Could you check a few things on this model? Use its own coordinates, in mm. Face numbers are marked on the shaded views. A direction names the side the tool comes from. Give positions to 0.01 mm unless a question says otherwise; leave off trailing zeros. Loops run counter-clockwise (first coordinate to the right, second up) from the corner with the lowest first, then second, coordinate; pieces in that order, holes last. Notation, with made-up numbers: (-23, 57) - (-10, 57) arc R16 cw to (-10, 61) - close; hole circle Ø3 at (7, 55.25). An arc over 180 degrees is marked (long way). One line per item, written item: value. Start each with the question number.
Q1. I'm going to push flat-ended pins straight in: P1, Ø10, axis at y = 13, z = 50, coming from the +X side; P2, Ø5, axis at y = 62.5, z = 36.5, coming from the -X side; P3, Ø13, axis at x = -20, z = 52.49, coming from the +Y side. Where does each tip first touch, or does it pass through?
Q2. I want a section at B-B (z = 22). Please give me the cut outline in (x, y), then the cut area to 3 significant figures.
Q3. If we mould it in two halves opening along Y, with no side actions, what happens to the marked faces 4, 5 and 6? For each: released by +Y, released by -Y, zero draft, split by the parting line, or undercut.
Q4. For the marked faces 1, 2 and 3, which set-ups out of +Z, -Z, +X, -X, +Y, -Y let a thin tool reach every point of the face, with its end or its side?
Q5. I want a section at D-D (z = 51). Please give me the cut outline in (x, y), then the cut area to 3 significant figures.
Q6. I want a section at C-C (x = -20). Please give me the cut outline in (y, z).
Q7. If I drill on line 1 (Y direction, x = -53.5, z = 24.5); line 2 (Z direction, x = 16, y = 14.5); line 3 (X direction, y = 10.5, z = 38), over which ranges is the centre line in solid material (lowest first)? Write a range as from..to.
Q8. I want a section at A-A (x = -68). Please give me the cut outline in (y, z), then the cut area to 3 significant figures.
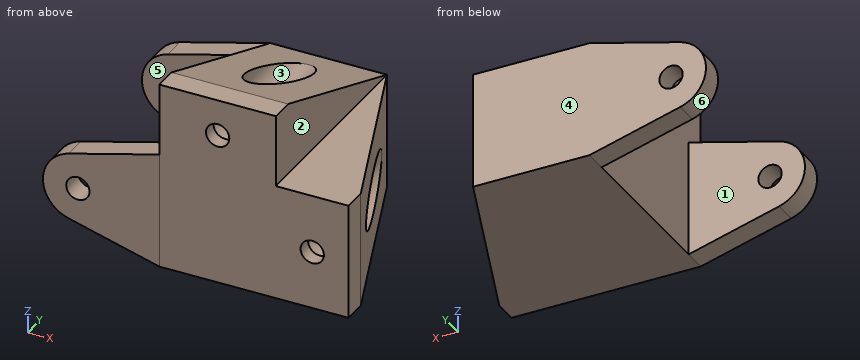
```python
from build123d import *

# Parameters (mm, degrees)
BOSS_EXTRUDE1_DEPTH = 40
BOSS_EXTRUDE2_DEPTH = 73.391828
SKETCH4_W           = 40
SKETCH4_H           = 57.391828437
CUT_EXTRUDE1_DEPTH  = 73
BOSS_EXTRUDE4_DEPTH = 40
SKETCH8_R           = 4
CUT_EXTRUDE2_DEPTH  = 127.52479018
SKETCH10_R          = 7.5
CUT_EXTRUDE3_DEPTH  = 124.691569016


with BuildPart() as part:
    # Sketch2 → Boss-Extrude1 (new body)
    with BuildSketch(Plane.XY):
        Polygon((0, 0), (-40, 0), (-40, 73.391828437), (0, 73.391828437), (24.978165939, 8), (24.978165939, 0), align=None)
    extrude(amount=BOSS_EXTRUDE1_DEPTH)

    # Sketch3 → Boss-Extrude2 (add)
    with BuildSketch(Plane(origin=(0, 73.391828437, 0), x_dir=(1, 0, 0), z_dir=(0, 1, 0))):
        with BuildLine():
            Line((-40, -40), (-71.131560336, -31.584184471))
            ThreePointArc((-71.131560336, -31.584184471), (-80, -20), (-71.131560336, -8.415815529))
            Line((-71.131560336, -8.415815529), (-40, 0))
            Line((-40, 0), (-40, -40))
        make_face()
    extrude(amount=-BOSS_EXTRUDE2_DEPTH)

    # Sketch4 → Cut-Extrude1 (cut)
    with BuildSketch(Plane.XY):
        with Locations((-60, 36.695914219)):
            Rectangle(SKETCH4_W, SKETCH4_H)
    extrude(amount=CUT_EXTRUDE1_DEPTH, mode=Mode.SUBTRACT)

    # Sketch6 → Boss-Extrude4 (add)
    with BuildSketch(Plane(origin=(0, 0, 0), x_dir=(0, 0, -1), z_dir=(1, 0, 0))):
        Polygon((-40, 73.391828437), (-64.978165939, 8), (-64.978165939, 0), (-40, 0), align=None)
    extrude(amount=-BOSS_EXTRUDE4_DEPTH)

    # Sketch8 → Cut-Extrude2 (cut, through all)
    with BuildSketch(Plane(origin=(0, 73.391828437, 0), x_dir=(1, 0, 0), z_dir=(0, 1, 0))):
        with Locations(Location((12.489082969, -20, 0), (0, 0, 270))):
            Circle(SKETCH8_R)
        with Locations(Location((-20, -52.489082969, 0), (0, 0, 270))):
            Circle(SKETCH8_R)
        with Locations(Location((-68, -20, 0), (0, 0, 270))):
            Circle(SKETCH8_R)
    extrude(amount=-CUT_EXTRUDE2_DEPTH, mode=Mode.SUBTRACT)

    # Sketch10 → Cut-Extrude3 (cut, through all)
    with BuildSketch(Plane(origin=(0, 5, 0), x_dir=(1, 0, 0), z_dir=(0, 1, 0))):
        with Locations((12.489082969, -20)):
            Circle(SKETCH10_R)
        with Locations(Location((-20, -52.489082969, 0), (0, 0, 270))):
            Circle(SKETCH10_R)
    extrude(amount=CUT_EXTRUDE3_DEPTH, mode=Mode.SUBTRACT)


solid = part.part
```
Worked answers:
1. P1: stops at x = 0
1. P2: stops at x = -40
1. P3: stops at y = 5
2. outline: (-79.83, 0) - (-71.46, 0) - (-71.46, 8) - (-79.83, 8) - close; (-79.83, 65.39) - (-71.46, 65.39) - (-71.46, 73.39) - (-79.83, 73.39) - close; (-64.54, 0) - (9.02, 0) - (9.02, 5) - (5.26, 5) - (5.26, 59.62) - (0, 73.39) - (-64.54, 73.39) - (-64.54, 65.39) - (-40, 65.39) - (-40, 8) - (-64.54, 8) - close; (15.95, 0) - (24.98, 0) - (24.98, 8) - (19.72, 21.77) - (19.72, 5) - (15.95, 5) - close
2. area: 3,930 mm²
3. face 4: released by +Y
3. face 5: undercut
3. face 6: zero draft
4. face 1: +Z, -Z, -X
4. face 2: +Z, +X, +Y, -Y
4. face 3: +Y
5. outline: (-40, 0) - (-23.71, 0) - (-23.71, 5) - (-27.35, 5) - (-27.35, 44.59) - (-40, 44.59) - close; (-16.29, 0) - (0, 0) - (0, 44.59) - (-12.65, 44.59) - (-12.65, 5) - (-16.29, 5) - close
5. area: 1,160 mm²
6. outline: (0, 0) - (73.39, 0) - (73.39, 40) - (60.33, 44.99) - (5, 44.99) - (5, 48.49) - (0, 48.49) - close; (0, 56.49) - (5, 56.49) - (5, 59.99) - (21.06, 59.99) - (8, 64.98) - (0, 64.98) - close
7. line 1: y = 0..8, 65.39..73.39
7. line 2: z = 0..13.37, 26.63..40
7. line 3: x = -40..24.02
8. outline: (0, 7.57) - (8, 7.57) - (8, 16) - (0, 16) - close; (0, 24) - (8, 24) - (8, 32.43) - (0, 32.43) - close; (65.39, 7.57) - (73.39, 7.57) - (73.39, 16) - (65.39, 16) - close; (65.39, 24) - (73.39, 24) - (73.39, 32.43) - (65.39, 32.43) - close
8. area: 270 mm²
